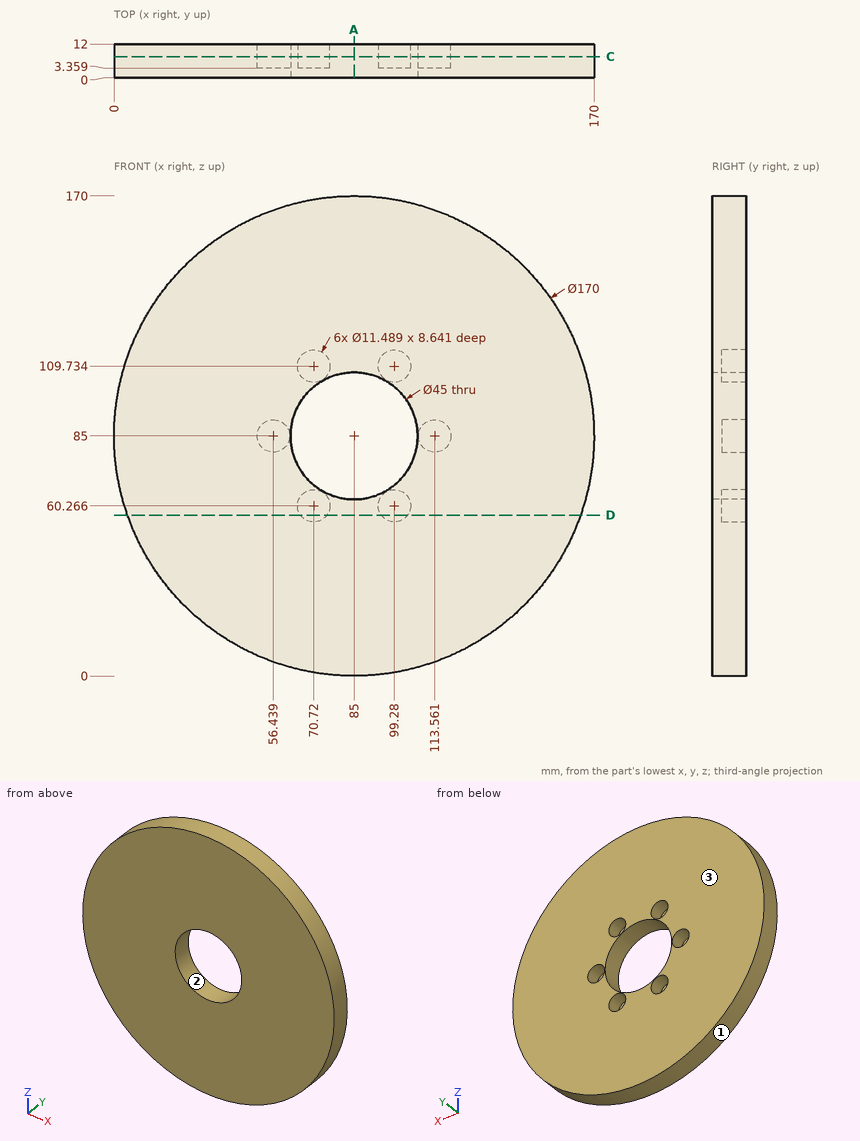
Print and shaded views of the part. All mm, measured from the part's lowest x, y and z. Coordinates: 2 decimals unless noted, no trailing zeros. Write each loop counter-clockwise with the first axis right and the second up, starting at its lowest first coordinate (ties: lowest second). Pieces come first, ordered by that corner, then holes. Notation, with made-up numbers: M 66,-38.5 L 124,-38.5 A9 ccw 124,-33.5 Z; hole C 88,-22.75 d6. An arc over 180 degrees is marked long. Return JSON: item names as keys, results as strings.
1. Saw through at A-A, the plane x = 85. Write the cut outline in (y, z), then the cut area to 3 significant figures.
Determined:
{"outline": "M 0,0 L 12,0 L 12,62.5 L 0,62.5 Z; M 0,107.5 L 12,107.5 L 12,170 L 0,170 Z", "area": "1,500 mm²"}
2. Pull direction X, two halves, no side cores. Call the marked faces 1, 2 and 3: pulls with the +X half, pulls with the -X half, needs draft (parallel to the pull), parting line crosses it, or undercut.
Determined:
{"face 1": "parting line crosses it", "face 2": "undercut", "face 3": "needs draft"}
3. Saw through at D-D, the plane z = 57. Write the cut outline in (x, y) (1 decimal), then the cut area to 3 significant figures.
Determined:
{"outline": "M 4.7,0 L 165.3,0 L 165.3,12 L 104,12 L 104,3.4 L 94.6,3.4 L 94.6,12 L 75.4,12 L 75.4,3.4 L 66,3.4 L 66,12 L 4.7,12 Z", "area": "1,760 mm²"}
4. Probe L1, parallel to X at y = 6.25, z = 85 (1 decimal); L2, parallel to X at y = 5.5, z = 56.5; L3, parallel to X at y = 9, z = 82. List the from-to ranges inside material, lowest first.
Determined:
{"L1": "0 to 50.7, 62.2 to 62.5, 107.5 to 107.8, 119.3 to 170", "L2": "4.92 to 66.38, 75.06 to 94.94, 103.62 to 165.08", "L3": "0.05 to 51.54, 61.34 to 62.7, 107.3 to 108.66, 118.46 to 169.95"}
5. Flat gauge pins, fed straight in: pin 1 Ø7 at (x, z) = (99.28, 109.73) entering from +Y; pin 2 Ø1 at (y, z) = (10, 22.5) entering from -X (1 decimal); pin 3 Ø1 at (y, z) = (10.5, 58) entering from -X. Where does each tip first touch, or does it go through?
Determined:
{"pin 1": "y = 3.36", "pin 2": "x = 26.9", "pin 3": "x = 4.24"}
6. Saw through at C-C, the plane y = 7.5. Write the cut outline in (x, z) (1 decimal), then the cut area to 3 significant figures.
Determined:
{"outline": "C 85,85 d170; hole C 56.4,85 d11.5; hole C 85,85 d45; hole C 70.7,60.3 d11.5; hole C 70.7,109.7 d11.5; hole C 99.3,60.3 d11.5; hole C 99.3,109.7 d11.5; hole C 113.6,85 d11.5", "area": "20,500 mm²"}
